The figure shows three views and two pictorial views of one solid part (mm, origin at its lowest corner). Answer the questions. A direction names the side the tool comes from. Coordinates: 2 decimals unless noted, no trailing zeros. Order: outer loops, then holes, each group sorted by start corner. A loop starts at its lowest first (then second) coordinate and runs counter-clockwise, first axis right, second up. Notation, with made-up numbers: M 3.25,66 L 7.25,66 A21 ccw 7.25,98 Z; hole C 72.25,35.25 d6. An arc over 180 degrees is marked long. Answer in a Markdown table with one row per item. Add a question column.
Item 1: The mould has two halves that part along Z. Classify the marked faces 1, 2 and 3: released by +Z, released by -Z, zero draft, split by the parting line, or undercut.
Item 2: The part is cut by section A-A (y = 5.75). State how many separate pieces and enclosed holes the cut face has, then the cut area to 3 significant figures.
Item 3: The part is cut by section C-C (x = 16). Write down the section's boundary in (y, z).
Item 4: Which of the six approach directions +Z, -Z, +X, -X, +Y, -Y give full straight-line access (tool end or side, diameter ignored) to the marked faces 4, 5, 6, 7 and 8?
Item 5: Consider line 1 (Z direction, x = 48.5, y = 5.25) (1 decimal); line 2 (X direction, y = 2, z = 89.5). Determine where each line is inside the solid, lowest interval first. Write a range as from..to.
Item 6: The part is cut by section D-D (z = 82.5). Write down the section's boundary in (x, y), then the cut area to 3 significant figures.
Item 7: Flat-ended cylindrical pins translate along their axes: pin 1 Ø4 at (y, z) = (6.5, 11.5) entering from +X; pin 2 Ø2 at (y, z) = (2, 72) entering from -X; pin 3 Ø4 at (x, y) = (74, 3.5) entering from +Z; pin 4 Ø3 at (x, z) = (48.33, 92.33) entering from -Y. Find the tip coordinate at first contact, or state that the pin passes through.
Item 8: The part is cut by section B-B (x = 40.5). Write down the section's boundary in (y, z), then the cut area to 3 significant figures.
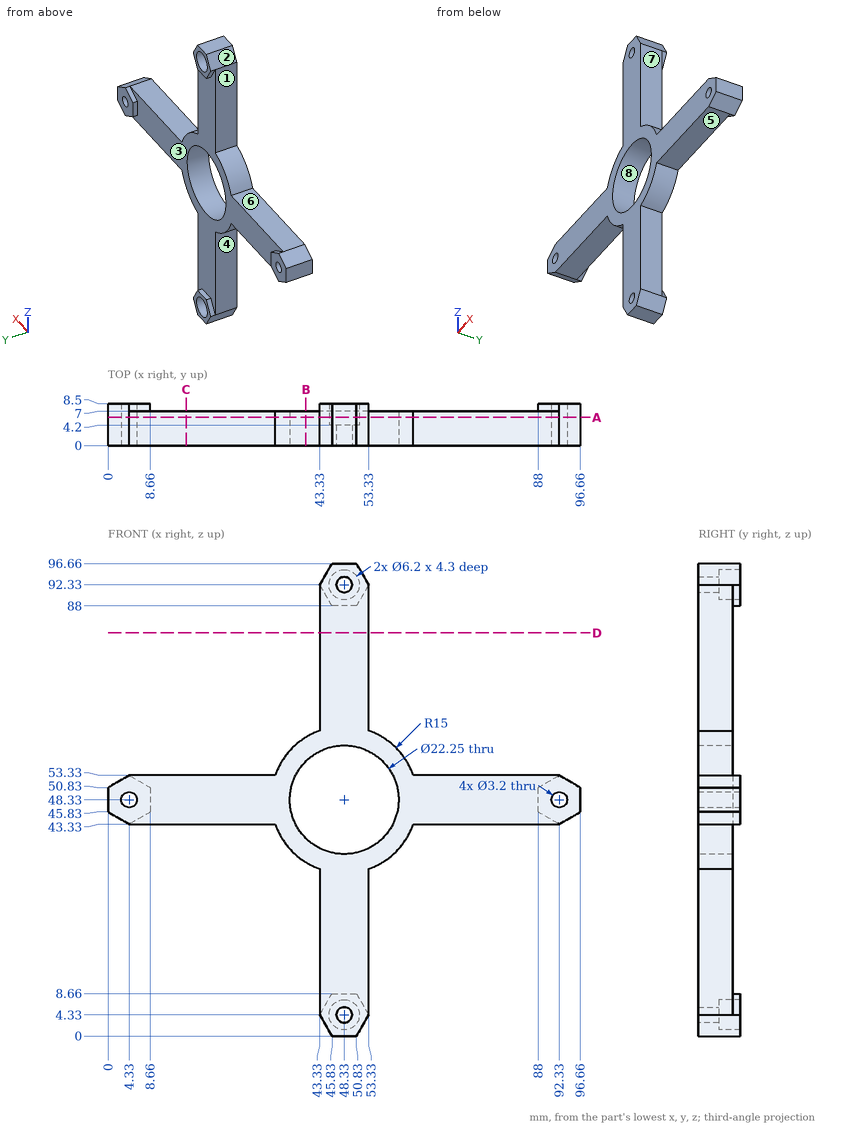
Reply:
| question | item | result |
|---|---|---|
| 1 | face 1 | zero draft |
| 1 | face 2 | released by +Z |
| 1 | face 3 | undercut |
| 2 | separate pieces | 1 |
| 2 | enclosed holes | 5 |
| 2 | area | 1,540 mm2 |
| 3 | outline | M 0,43.33 L 7,43.33 L 7,53.33 L 0,53.33 Z |
| 4 | face 4 | -Z, -X, +Y, -Y |
| 4 | face 5 | -Z, +X, +Y, -Y |
| 4 | face 6 | +Z, -X, +Y, -Y |
| 4 | face 7 | +Z, +X, +Y, -Y |
| 4 | face 8 | +Y, -Y |
| 5 | line 1 | z = 0..1.2, 7.4..37.2, 59.5..89.2, 95.4..96.7 |
| 5 | line 2 | x = 43.33..53.33 |
| 6 | outline | M 43.33,0 L 53.33,0 L 53.33,7 L 43.33,7 Z |
| 6 | area | 70.0 mm2 |
| 7 | pin 1 | stops at x = 53.33 |
| 7 | pin 2 | stops at x = 43.33 |
| 7 | pin 3 | stops at z = 53.33 |
| 7 | pin 4 | passes through |
| 8 | outline | M 0,35.54 L 7,35.54 L 7,40.43 L 0,40.43 Z; M 0,56.23 L 7,56.23 L 7,61.12 L 0,61.12 Z |
| 8 | area | 68.5 mm2 |
